The listing builds one solid part. Answer for the finished solid, in the listing's coordinates (mm). Give positions to 0.01 mm unless a question says otherwise; leave off trailing zeros. Order: outer loops, then holes, each group sorted by start corner. A loop starts at its lowest first (then second) coordinate and runs counter-clockwise, first axis right, second up. Notation, with made-up numbers: (-10, -38.5) - (13, -38.5) arc R20 cw to (13, -15.5) - close; hole circle Ø10 at (60.5, 23). An arc over 180 degrees is marked (long way). Use a Markdown table: item, result. Add a question column.
1) Find section A-A, the plane x = 0. Determine the outline of the cut face in (y, z) (3 decimals), plus the area to 3 significant figures.
2) Flat-ended cylindrical pins translate along their axes: pin 1 (1 mm diameter, centred on x = 4, z = -2, fed in from -Y); pin 2 (2 mm diameter, centred on x = -2, z = 1.5, fed in from -Y) (3 decimals); pin 3 (1 mm diameter, centred on y = 1, z = 3, fed in from +X). Find the tip coordinate at first contact, or state that the pin passes through.
3) Straight lines are drawn through the part: line 1 (Z direction, x = 0, y = 2.2) (3 decimals); line 2 (Z direction, x = -2.75, y = 0.3); line 3 (X direction, y = 1.7, z = -1.75). For each, find the intervals that lie inside material, in ascending order.
4) Find section B-B, the plane y = 1.7. Determine the outline of the cut face in (x, z) (3 decimals), plus the area to 3 significant figures.
5) The mould has two halves that part along Z. Classify faces 1 (the face through (4.8, 2.8, -2.8)), 2 (the face through (0, 3, 5.555)), 3 (the face through (0.69, 2.84, 3.1)): released by +Z, released by -Z, zero draft, split by the parting line, or undercut.
6) Find section C-C, the plane y = 5.3. Determine the outline of the cut face in (x, z) (3 decimals).
Autodesk Inventor part; units mm, degrees
ref_plane "YZ Plane" through (0, 0, 0) normal (1, 0, 0) x (0, 1, 0)
ref_plane "XZ Plane" through (0, 0, 0) normal (0, 1, 0) x (-1, 0, 0)
ref_plane "XY Plane" through (0, 0, 0) normal (0, 0, 1) x (1, 0, 0)
sketch "Esboço1" plane through (0, 0, 0) normal (0, 1, 0) x (-1, 0, 0)
  circle A0 centre (0, 0) radius 3.175
  line L0 (-3.2072, -5.555) -> (-6.4144, 0)
  line L1 (-6.4144, 0) -> (-3.2072, 5.555)
  line L2 (-3.2072, 5.555) -> (3.2072, 5.555)
  line L3 (3.2072, 5.555) -> (6.4144, 0)
  line L4 (6.4144, 0) -> (3.2072, -5.555)
  line L5 (3.2072, -5.555) -> (-3.2072, -5.555)
  dimension "d0" = 6.35
extrude "Extrusão1" add sketch "Esboço1" along normal blind 5.74
thread "Rosca1"
sketch "Esboço2" plane through (0, 0, 0) normal (0, 0, 1) x (1, 0, 0)
  line L0 (0, 0) -> (-3.175, 0)
  line L1 (3.2072, 5.74) -> (-3.2072, 5.74)
  line L2 (-3.2072, 5.74) -> (-6.4144, 5.74)
  line L3 (0, 0) -> (0, 10.6611)
  line L4 (-6.4144, 4.74) -> (-5.4144, 5.74)
  line L5 (-3.175, 4.99) -> (-3.925, 5.74)
  line L6 (-3.2072, 2.87) -> (-11.6119, 2.87)
  line L7 (-6.4144, 4.74) -> (-6.4144, 5.74)
  line L8 (-6.4144, 5.74) -> (-5.4144, 5.74)
  line L9 (-3.925, 5.74) -> (-3.175, 5.74)
  line L10 (-3.175, 4.99) -> (-3.175, 5.74)
  line L11 (-3.2072, 0) -> (-6.4144, 0)
  line L12 (-6.4144, 1) -> (-5.4144, 0)
  line L13 (-3.175, 0.75) -> (-3.925, 0)
  line L14 (-6.4144, 1) -> (-6.4144, 0)
  line L15 (-6.4144, 0) -> (-5.4144, 0)
  line L16 (-3.925, 0) -> (-3.175, 0)
  line L17 (-3.175, 0.75) -> (-3.175, 0)
  line L18 (-6.4144, 0) -> (-3.2072, 0)
  line L19 (-6.4144, 0) -> (-5.4144, 0)
  point P0 (-3.175, 5.74)
  dimension "d6" = 1
  dimension "d7" = 1
  dimension "d8" = 0.75
  dimension "d9" = 0.75
revolve "Revolução1" cut sketch "Esboço2" angle 360 about axis through (0, 0, 0) along (0, 1, 0)
equation "\"d7\" = d6"
equation "\"d9\" = d8"
properties part number "Porca sextavada 1 quarto" material "Aço, carbono"
The answers:
| question | item | result |
|---|---|---|
| 1 | outline | (0, -5.414) - (0.141, -5.555) - (5.599, -5.555) - (5.74, -5.414) - (5.74, -3.925) - (4.99, -3.175) - (0.75, -3.175) - (0, -3.925) - close; (0, 3.925) - (0.75, 3.175) - (4.99, 3.175) - (5.74, 3.925) - (5.74, 5.414) - (5.599, 5.555) - (0.141, 5.555) - (0, 5.414) - close |
| 1 | area | 26.2 mm2 |
| 2 | pin 1 | y = 0 |
| 2 | pin 2 | y = 0.425 |
| 2 | pin 3 | x = 4.97 |
| 3 | line 1 | -5.555 to -3.175, 3.175 to 5.555 |
| 3 | line 2 | -5.01 to -2.36, 2.36 to 5.01 |
| 3 | line 3 | -5.4 to -2.65, 2.65 to 5.4 |
| 4 | outline | (-6.414, 0) - (-3.207, -5.555) - (3.207, -5.555) - (6.414, 0) - (3.207, 5.555) - (-3.207, 5.555) - close; hole circle Ø6.35 at (0, 0) |
| 4 | area | 75.2 mm2 |
| 5 | face 1 | released by -Z |
| 5 | face 2 | released by +Z |
| 5 | face 3 | undercut |
| 6 | outline | (-5.735, -1.177) - (-3.887, -4.378) arc R5.854 ccw to (-1.848, -5.555) - (1.848, -5.555) arc R5.854 ccw to (3.887, -4.378) - (5.735, -1.177) arc R5.854 ccw to (5.735, 1.177) - (3.887, 4.378) arc R5.854 ccw to (1.848, 5.555) - (-1.848, 5.555) arc R5.854 ccw to (-3.887, 4.378) - (-5.735, 1.177) arc R5.854 ccw to start; hole circle Ø6.97 at (0, 0) |
